The listing builds one solid part. Answer for the finished solid, in the listing's coordinates (mm). Coordinates: 2 decimals unless noted, no trailing zeros. Loops run counter-clockwise (first coordinate to the right, second up) from the corner with the lowest first, then second, coordinate; pieces in that order, holes last. Notation, with made-up numbers: (25.25, -6.5) - (50.25, -6.5) arc R24 cw to (50.25, 12.5) - close; hole circle Ø10 at (25, 13). An arc over 180 degrees is marked (long way). Return JSON: item names as keys, results as strings. Group by question number.
1. Find the intervals of material crossed by line 1 along Z through (x, y) = (-18, 4.5); line 2 along X through (y, z) = (1, -32.5); line 3 along X through (y, z) = (5.5, -75.5), in increasing order.
2. Section D-D (z = -32.75) is taken. Write down the section's boundary in (x, y), and give its area (3 significant figures).
3. This flat-tipped pin is pushed along its axis until it touches: P1, Ø4, axis at x = -18, z = -9.5, coming from the -Y side. Where does it stop, or does it pass through?
4. Section C-C (x = -18) is taken. Write down the section's boundary in (y, z).
5. The mould has two halves that part along X. Classify faces 1 (the face through (0, 5, -51)), 2 (the face through (-80, 5, -49)), 3 (the face through (-55.806, 4.93, -26.265)), 4 (the face through (-41, 5, -100)): pulls with the +X half, pulls with the -X half, needs draft (parallel to the pull), parting line crosses it, or undercut.
6. Section B-B (y = 8.75) is taken. Write down the section's boundary in (x, z), and give its area (3 significant figures).
7. Section A-A (z = -9.5) is taken. Write down the section's boundary in (x, y).
Autodesk Inventor part; units mm, degrees
ref_plane "YZ Plane" through (0, 0, 0) normal (1, 0, 0) x (0, 1, 0)
ref_plane "XZ Plane" through (0, 0, 0) normal (0, 1, 0) x (-1, 0, 0)
ref_plane "XY Plane" through (0, 0, 0) normal (0, 0, 1) x (1, 0, 0)
sketch "Sketch1" plane through (0, 0, 0) normal (0, 1, 0) x (-1, 0, 0)
  line L0 (0, 0) -> (80, 0)
  line L1 (80, 0) -> (80, -100)
  line L2 (80, -100) -> (0, -100)
  line L3 (0, -100) -> (0, 0)
  line L4 (55, 12.5326) -> (55, -107.8943) construction
  circle A0 centre (55, -25) radius 1.5
  circle A1 centre (55, -75) radius 1.5
  line L5 (55, -25) -> (18, -25) construction
  circle A2 centre (18, -25) radius 1.5
  circle A3 centre (18, -25) radius 6.25
  circle A4 centre (18, -9.5) radius 1.5
  circle A5 centre (4.5766, -32.75) radius 1.5
  circle A6 centre (31.4234, -32.75) radius 1.5
  dimension "d2" = 25
  dimension "d3" = 3
  dimension "d4" = 3
  dimension "d5" = 25
  dimension "d6" = 50
  dimension "d7" = 37
  dimension "d8" = 3
  dimension "d9" = 100
  dimension "d10" = 80
  dimension "d13" = 12.5
  dimension "d16" = 3
  dimension "d17" = 15.5
  dimension "d20" = 360
  dimension "d22" = 12.5326
  dimension "d23" = 107.8943
  dimension "d27" = 48.5766
extrude "Extrusion1" add sketch "Sketch1" along normal blind 10 contours L0 L1 L2 L3 | A3 | A4 | A5 | A6
extrude "Extrusion2" cut sketch "Sketch1" along normal blind 10 contours A3
extrude "Extrusion3" cut sketch "Sketch1" along normal blind 10 contours A4 | A5 | A6
properties part number "Support test1"
The answers:
{
 "1": {"line 1": "z = -100 to -31.25, -18.75 to -11, -8 to 0", "line 2": "x = -80 to -32.9, -29.94 to -6.06, -3.1 to 0", "line 3": "x = -80 to -56.41, -53.59 to 0"},
 "2": {"outline": "(-80, 0) - (-32.92, 0) - (-32.92, 10) - (-80, 10) - close; (-29.92, 0) - (-6.08, 0) - (-6.08, 10) - (-29.92, 10) - close; (-3.08, 0) - (0, 0) - (0, 10) - (-3.08, 10) - close", "area": "740 mm2"},
 "3": {"P1": "stops at y = 0"},
 "4": {"outline": "(0, -100) - (10, -100) - (10, -31.25) - (0, -31.25) - close; (0, -18.75) - (10, -18.75) - (10, -11) - (0, -11) - close; (0, -8) - (10, -8) - (10, 0) - (0, 0) - close"},
 "5": {"face 1": "pulls with the +X half", "face 2": "pulls with the -X half", "face 3": "undercut", "face 4": "needs draft"},
 "6": {"outline": "(-80, -100) - (0, -100) - (0, 0) - (-80, 0) - close; hole circle Ø3 at (-55, -75); hole circle Ø3 at (-55, -25); hole circle Ø3 at (-31.42, -32.75); hole circle Ø12.5 at (-18, -25); hole circle Ø3 at (-18, -9.5); hole circle Ø3 at (-4.58, -32.75)", "area": "7,840 mm2"},
 "7": {"outline": "(-80, 0) - (-19.5, 0) - (-19.5, 10) - (-80, 10) - close; (-16.5, 0) - (0, 0) - (0, 10) - (-16.5, 10) - close"}
}
